from build123d import *

# Parameters (mm, degrees)
SKETCH3_R          = 10
SKETCH3_R_2        = 5
CUT_EXTRUDE1_DEPTH = 73.756443014


with BuildPart() as part:
    # Sketch2 → Revolve1 (revolve)
    with BuildSketch(Plane(origin=(0, 0, 0), x_dir=(0, 0, -1), z_dir=(1, 0, 0)), mode=Mode.PRIVATE) as revolve1_sk:
        Polygon((-17.5, 42.5), (17.5, 42.5), (17.5, 38), (5.5, 35), (5.5, 18), (20.5, 16), (20.5, 0), (-20.5, 0), (-20.5, 16), (-5.5, 18), (-5.5, 35), (-17.5, 38), align=None)
    revolve(revolve1_sk.sketch.rotate(Axis((0, 0, 152.018729057), (0, 0, -1)), 90), axis=Axis((0, 0, 152.018729057), (0, 0, -1)))

    # Sketch3 → Cut-Extrude1 (cut, through all)
    with BuildSketch(Plane.XY.offset(20.5)):
        Circle(SKETCH3_R)
        with Locations((0, 26.5)):
            Circle(SKETCH3_R_2)
        with Locations((26.5, 0)):
            Circle(SKETCH3_R_2)
        with Locations((0, -26.5)):
            Circle(SKETCH3_R_2)
        with Locations((-26.5, 0)):
            Circle(SKETCH3_R_2)
    extrude(amount=-CUT_EXTRUDE1_DEPTH, mode=Mode.SUBTRACT)


solid = part.part
Here's how the part is built. I have some questions about the finished solid (model axes, mm). A direction names the side the tool comes from. Coordinates: 2 decimals unless noted, no trailing zeros. Write each loop counter-clockwise with the first axis right and the second up, starting at its lowest first coordinate (ties: lowest second). Pieces come first, ordered by that corner, then holes.
1) Thinking about a two-plate mould opening in Y: for faces 3 (the face through (-3.634, 16.365, -14.772)), 4 (the face through (40.537, -12.766, -0.245)), 5 (the face through (32, 22, 17.5)), 6 (the face through (-15, 15, 5.5)), which applies, +Y half, -Y half, draft (parallel to the pull), parting line (faces both ways), or undercut?
Filled in:
face 3: undercut
face 4: parting line
face 5: draft
face 6: undercut
2) If we section it at A-A (y = 0): Count the separate pieces of the cut face and the enclosed holes in it, plus the area to 3 significant figures.
Filled in:
separate pieces: 4
enclosed holes: 0
area: 1,200 mm2
3) If we section it at C-C (z = -14): List the corners of the cut face in (x, y) for me (3 decimals), plus the area to 3 significant figures.
Filled in:
outline: circle Ø85 at (0, 0); circle Ø33.733 at (0, 0); hole circle Ø74.25 at (0, 0); hole circle Ø20 at (0, 0)
area: 1,920 mm2
4) If we section it at B-B (z = 1.5): List the corners of the cut face in (x, y) for me.
Filled in:
outline: circle Ø85 at (0, 0); hole circle Ø10 at (-26.5, 0); hole circle Ø20 at (0, 0); hole circle Ø10 at (0, -26.5); hole circle Ø10 at (0, 26.5); hole circle Ø10 at (26.5, 0)
5) Which directions (+Z, -Z, +X, -X, +Y, -Y) give clear straight access to the entire face, cutting with the end or side of a thin tool? Please do faces 1 (the face through (15, 15, -5.5)), 2 (the face through (-10.4, -0.2, 20.5)).
Filled in:
face 1: -Z
face 2: +Z, +X, -X, +Y, -Y
6) If I drill on line 1 (Y direction, x = 0, z = -2); line 2 (Y direction, x = 7.5, z = -11.5); line 3 (X direction, y = 2.5, z = 12), over which ranges is the centre line in solid material (lowest first)?
Filled in:
line 1: y = -42.5 to -31.5, -21.5 to -10, 10 to 21.5, 31.5 to 42.5
line 2: y = -41.83 to -35.72, -15.48 to -6.61, 6.61 to 15.48, 35.72 to 41.83
line 3: x = -42.43 to -36.54, -16.95 to -9.68, 9.68 to 16.95, 36.54 to 42.43
7) I'm going to push flat-ended pins straight in: pin 1 (13 mm diameter, centred on x = 0, y = -26.5, fed in from -Z); pin 2 (10 mm diameter, centred on x = -5.5, z = 15.5, fed in from +Y); pin 3 (11.5 mm diameter, centred on x = 26.5, y = 0, fed in from +Z). Where does each tip first touch, or does it pass through?
Filled in:
pin 1: stops at z = -5.5
pin 2: stops at y = 42.5
pin 3: stops at z = 5.5
